Design review of the part built by this model. Coordinates are the model's own, in mm. A direction names the side the tool comes from. Coordinates: 2 decimals unless noted, no trailing zeros. Loops run counter-clockwise (first coordinate to the right, second up) from the corner with the lowest first, then second, coordinate; pieces in that order, holes last. Notation, with made-up numbers: M 62.25,53 L 118.25,53 A23 ccw 118.25,84 Z; hole C 59.25,-6.75 d10. An arc over 180 degrees is marked long. Answer as a JSON object with one key per item and string values. Group by question number.
1. To check wall thickness, follow probe 1 along Y at (x, z) = (19.5, 0.25); probe 2 along X at (y, z) = (14.75, -1.3); probe 3 along Z at (x, y) = (89, 14). State the ranges of each line that lie inside material, in increasing order.
2. Consider section C-C (z = -1.3). State the section outline as (x, y) points.
3. Draft analysis for pull direction X (two halves, no side actions). For faces 1 (the flat face through (46, 0, 1)), 2 (the flat face through (20, 21, 2)), 3 (the flat face through (84, 5, 1)), state which applies: +X half, -X half, draft (parallel to the pull), parting line (faces both ways), or undercut.
4. Insertion check: pin 1 (5 mm diameter, centred on x = 73, y = 25.5, fed in from -Z); pin 2 (0.9 mm diameter, centred on y = 26, z = 1, fed in from +X); pin 3 (3 mm diameter, centred on x = 9.5, y = 14, fed in from +Z). Each pin has a flat end and moves straight along its axis. Give the tip position at first contact, or say it passes through.
5. Consider section A-A (y = 15). State the section outline as (x, z) points.
6. Consider section D-D (y = 11.5). State the section outline as (x, z) points.
7. Consider section B-B (x = 21). State the section outline as (y, z) points.
8. Machinability: for faces 4 (the flat face through (43, 15, 3)), 5 (the flat face through (84, 25, 1)), 6 (the cylindrical face through (31, 15, 2)), which of the approach directions +Z, -Z, +X, -X, +Y, -Y give a long, thin tool a straight path to every point of the face, cutting with its end or side? Answer none if there is none.
from build123d import *

# Parameters (mm, degrees)
SKETCH_1_W               = 88
SKETCH_1_H               = 3
EXTRUDE_1_DEPTH          = 30
SKETCH_2_R               = 4.5
EXTRUDE_1_2_DEPTH        = 30
SKETCH_3_R               = 2.5
CUT_EXTRUDE_1_DEPTH      = 31
SKETCH_4_W               = 11
SKETCH_4_H               = 10.4
SKETCH_4_H_2             = 10
CUT_EXTRUDE_2_DEPTH      = 4.2
CUT_EXTRUDE_2_DEPTH_BACK = 6.8
CUT_EXTRUDE_3_DEPTH      = 9.8


with BuildPart() as part:
    # Эскиз1 → Extrude 1 (new body)
    with BuildSketch(Plane(origin=(0, 0, 0), x_dir=(1, 0, 0), z_dir=(0, 1, 0))):
        with Locations((44, -1.5)):
            Rectangle(SKETCH_1_W, SKETCH_1_H)
    extrude(amount=EXTRUDE_1_DEPTH)

    # Эскиз2 → Extrude 1 2 (add)
    with BuildSketch(Plane(origin=(0, 0, 0), x_dir=(1, 0, 0), z_dir=(0, 1, 0))):
        with Locations((89, 1.3)):
            Circle(SKETCH_2_R)
    extrude(amount=EXTRUDE_1_2_DEPTH)

    # Эскиз3 → Вырез-Вытянуть1 (cut, through all)
    with BuildSketch(Plane(origin=(0, 0, 0), x_dir=(1, 0, 0), z_dir=(0, 1, 0))):
        with Locations((89, 1.3)):
            Circle(SKETCH_3_R)
    extrude(amount=CUT_EXTRUDE_1_DEPTH, mode=Mode.SUBTRACT)

    # Эскиз4 → Вырез-Вытянуть2 (cut, two sides)
    with BuildSketch(Plane.XY) as cut_extrude_2_sk:
        with Locations((89.5, 24.8)):
            Rectangle(SKETCH_4_W, SKETCH_4_H)
        with Locations((89.5, 5)):
            Rectangle(SKETCH_4_W, SKETCH_4_H_2)
    extrude(amount=CUT_EXTRUDE_2_DEPTH, mode=Mode.SUBTRACT)
    extrude(cut_extrude_2_sk.sketch, amount=-CUT_EXTRUDE_2_DEPTH_BACK, mode=Mode.SUBTRACT)

    # Эскиз5 → Вырез-Вытянуть3 (cut, through all)
    with BuildSketch(Plane.XY.offset(3)):
        with BuildLine():
            Line((15, 21), (25, 21))
            ThreePointArc((25, 21), (31, 15), (25, 9))
            Line((25, 9), (15, 9))
            ThreePointArc((15, 9), (9, 15), (15, 21))
        make_face()
        with BuildLine():
            Line((10, 30), (0, 30))
            Line((0, 30), (0, 20))
            ThreePointArc((0, 20), (2.928932188, 27.071067812), (10, 30))
        make_face()
        with BuildLine():
            Line((0, 10), (0, 0))
            Line((0, 0), (10, 0))
            ThreePointArc((10, 0), (2.928932188, 2.928932188), (0, 10))
        make_face()
    extrude(amount=-CUT_EXTRUDE_3_DEPTH, mode=Mode.SUBTRACT)


solid = part.part
Findings below:
{
 "1": {"probe 1": "y = 0 to 9, 21 to 30", "probe 2": "x = 84.5 to 86.5, 91.5 to 93.5", "probe 3": "z = -5.8 to -3.8, 1.2 to 3.2"},
 "2": {"outline": "M 84.5,10 L 86.5,10 L 86.5,19.6 L 84.5,19.6 Z; M 91.5,10 L 93.5,10 L 93.5,19.6 L 91.5,19.6 Z"},
 "3": {"face 1": "draft", "face 2": "undercut", "face 3": "+X half"},
 "4": {"pin 1": "stops at z = 0", "pin 2": "stops at x = 84", "pin 3": "stops at z = 3"},
 "5": {"outline": "M 0,0 L 9,0 L 9,3 L 0,3 Z; M 31,0 L 84.69,0 A4.5 ccw long 87.67,3 L 31,3 Z; hole C 89,-1.3 d5"},
 "6": {"outline": "M 0,0 L 10.13,0 L 10.13,3 L 0,3 Z; M 29.87,0 L 84.69,0 A4.5 ccw long 87.67,3 L 29.87,3 Z; hole C 89,-1.3 d5"},
 "7": {"outline": "M 0,0 L 9,0 L 9,3 L 0,3 Z; M 21,0 L 30,0 L 30,3 L 21,3 Z"},
 "8": {"face 4": "+Z, -X, +Y, -Y", "face 5": "+Z, -Z, +X, +Y", "face 6": "+Z, -Z"}
}
